Print and shaded views of the part. All mm, measured from the part's lowest x, y and z. A direction names the side the tool comes from. Round coordinates to 2 decimals unless told otherwise and drop trailing zeros. Loops run counter-clockwise (first coordinate to the right, second up) from the corner with the lowest first, then second, coordinate; pieces in that order, holes last. Notation, with made-up numbers: (36, -21) -> (72, -21) arc R19 ccw to (72, -12) -> close; hole circle Ø6 at (37, 12). An arc over 180 degrees is marked (long way). Answer as CSV lines item,"result".
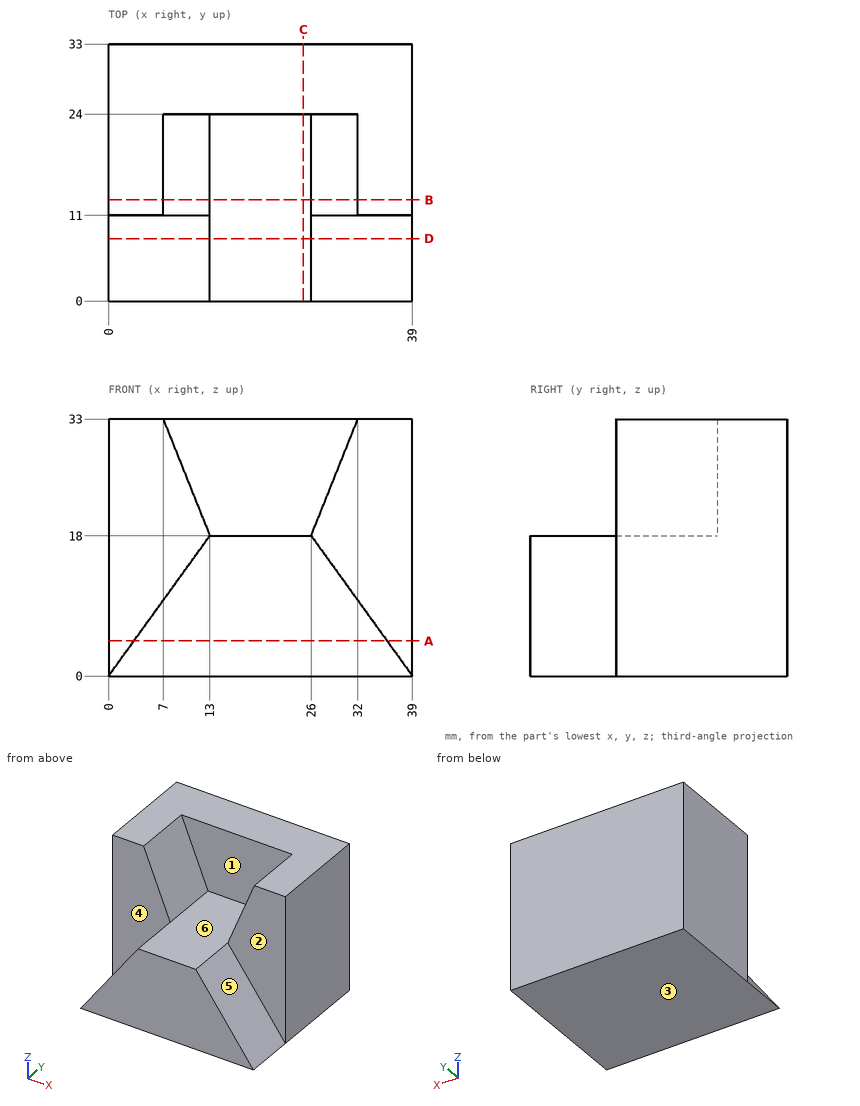
Q1. Probe L1, parallel to Y at x = 4, z = 26.5; L2, parallel to Y at x = 22, z = 27.5; L3, parallel to X at y = 23, z = 30.5. List the from-to ranges inside material, lowest first. Write a range as [from, to].
Results:
L1,"[11, 33]"
L2,"[24, 33]"
L3,"[0, 8], [31, 39]"
Q2. Two-plate mould, pull along X, no slides. Class the marked faces 4, 5 and 6: pulls with the +X half, pulls with the -X half, needs draft (parallel to the pull), parting line crosses it, or undercut.
Results:
face 4,"needs draft"
face 5,"pulls with the +X half"
face 6,"undercut"
Q3. Slice it at C-C, the plane x = 25. Give the cut face in (y, z).
Results:
outline,"(0, 0) -> (33, 0) -> (33, 33) -> (24, 33) -> (24, 18) -> (0, 18) -> close"
Q4. Slice it at D-D, the plane y = 8. Give the cut face in (x, z).
Results:
outline,"(0, 0) -> (39, 0) -> (26, 18) -> (13, 18) -> close"
Q5. Slice it at A-A, the plane z = 4.5. Give the cut face in (x, y).
Results:
outline,"(0, 11) -> (3.25, 11) -> (3.25, 0) -> (35.75, 0) -> (35.75, 11) -> (39, 11) -> (39, 33) -> (0, 33) -> close"
Q6. Slice it at B-B, the plane y = 13. Give the cut face in (x, z), and give its area (3 significant figures).
Results:
outline,"(0, 0) -> (39, 0) -> (39, 33) -> (32, 33) -> (26, 18) -> (13, 18) -> (7, 33) -> (0, 33) -> close"
area,"1,000 mm2"
Q7. Tool access for the marked faces 1, 2 and 3: list every direction of +Z, -Z, +X, -X, +Y, -Y with a clear straight run to the whole face (end or side of a thin tool).
Results:
face 1,"+Z, -Y"
face 2,"+Z, +X, -Y"
face 3,"-Z, +X, -X, +Y, -Y"
Q8. Drop flat-ended pins along their axis: pin 1 Ø12 at (x, z) = (18, 27) entering from -Y; pin 2 Ø6.5 at (x, z) = (30.5, 21) entering from -Y; pin 3 Ø4 at (x, y) = (21, 11.5) entering from +Z. Give the stop position or say it passes through.
Results:
pin 1,"y = 24"
pin 2,"y = 11"
pin 3,"z = 18"
